Geometry check sheet. Reference: the model listing, model coordinates, mm. A direction names the side the tool comes from. Round coordinates to 2 decimals unless told otherwise and drop trailing zeros. Order: outer loops, then holes, each group sorted by start corner. A loop starts at its lowest first (then second) coordinate and runs counter-clockwise, first axis right, second up.
```python
from build123d import *

# Parameters (mm, degrees)
F1_DEPTH = 20
F2_R     = 75
F3_DEPTH = 20.001
F4_R     = 5
F5_DEPTH = 20.001
F6_DEPTH = 25
F7_T     = -5


with BuildPart() as f1:
    # F0 (on Top) → F1 (new body)
    with BuildSketch(Plane.XY):
        Polygon((86.6025403784, -150), (173.2050807569, 0), (86.6025403784, 150), (-86.6025403784, 150), (-173.2050807569, 0), (-86.6025403784, -150), align=None)
    extrude(amount=F1_DEPTH)

    # F2 (on face) → F3 (cut, through all)
    with BuildSketch(Plane.XY.offset(20)):
        Circle(F2_R)
    extrude(amount=-F3_DEPTH, mode=Mode.SUBTRACT)

    # F4 (on face) → F5 (cut, through all)
    with BuildSketch(Plane.XY.offset(20)):
        with Locations((75, 129.9038105677)):
            Circle(F4_R)
        with Locations((-75, -129.9038105677)):
            Circle(F4_R)
        with Locations((-150, 0)):
            Circle(F4_R)
        with Locations((150, 0)):
            Circle(F4_R)
        with Locations((75, -129.9038105677)):
            Circle(F4_R)
    extrude(amount=-F5_DEPTH, mode=Mode.SUBTRACT)

    # F4 (on face) → F6 (cut)
    with BuildSketch(Plane.XY.offset(20)):
        with Locations((-75, 129.9038105677)):
            Circle(F4_R)
        with Locations((75, 129.9038105677)):
            Circle(F4_R)
        with Locations((-75, -129.9038105677)):
            Circle(F4_R)
        with Locations((-150, 0)):
            Circle(F4_R)
        with Locations((150, 0)):
            Circle(F4_R)
        with Locations((75, -129.9038105677)):
            Circle(F4_R)
    extrude(amount=-F6_DEPTH, mode=Mode.SUBTRACT)

    # F7
    f7_openings = [f1.faces().sort_by_distance(p)[0] for p in [
        (0, -145.417424, 0),
    ]]
    offset(amount=F7_T, openings=f7_openings)


solid = f1.part
```
(1) Draft check along Y on faces 3 (the flat face through (129.298, -76.05, 9.86)), 4 (the flat face through (23.3, 71.5, 0)), 5 (the cylindrical face through (-9.764, 74.362, 10.14)). Enter one of: released by +Y, released by -Y, zero draft, split by the parting line, or undercut.
Returned:
face 3: released by -Y
face 4: zero draft
face 5: undercut
(2) Material ranges on line 1 (X direction, y = -59, z = 2.75); line 2 (Y direction, x = -7, z = 4.75); line 3 (X direction, y = 53, z = 10.25), recorded low to high.
Returned:
line 1: x = -139.14 to -133.37, -54.03 to -46.3, 46.3 to 54.03, 133.37 to 139.14
line 2: y = -150 to -145, -79.69 to -74.67, 74.67 to 79.69, 145 to 150
line 3: x = -142.61 to -136.83, -59.92 to -53.07, 53.07 to 59.92, 136.83 to 142.61
(3) Sectioned sample at A-A, the plane z = 5. Give the number of separate pieces and of enclosed holes in the cut face, and give its area (3 significant figures).
Returned:
separate pieces: 8
enclosed holes: 8
area: 8,960 mm2
(4) Depth check by flat-ended pin: P1, Ø4, axis at y = -108.5, z = 2, coming from the -X side; P2, Ø3, axis at x = 131.5, z = 3.5, coming from the +Y side; P3, Ø1, axis at y = 119.5, z = 10, coming from the -X side; P4, Ø16, axis at x = -75, y = -129.9, coming from the +Z side. Enter the tip coordinate at first touch or a pass-through.
Returned:
P1: stops at x = -111.72
P2: stops at y = 74.83
P3: stops at x = -104.5
P4: stops at z = 20
(5) Sectioned sample at C-C, the plane y = 47.5. Record the cut outline in (x, z), and give its area (3 significant figures).
Returned:
outline: (-145.78, 0) - (-140.01, 0) - (-140.01, 15) - (-64.37, 15) - (-64.37, 0) - (-58.04, 0) - (-58.04, 20) - (-145.78, 20) - close; (58.04, 0) - (64.37, 0) - (64.37, 15) - (140.01, 15) - (140.01, 0) - (145.78, 0) - (145.78, 20) - (58.04, 20) - close
area: 1,240 mm2
(6) Set-up check for faces 1 (the cylindrical face through (67.63, 136.66, 7.6)), 2 (the flat face through (70, 128, 0)): record each of +Z, -Z, +X, -X, +Y, -Y from which the full face is reachable in a straight line by a thin tool's end or side.
Returned:
face 1: -Z
face 2: -Z, +X, -X, +Y, -Y
(7) Sectioned sample at B-B, the plane x = -150. Record the cut outline in (y, z), and give its area (3 significant figures).
Returned:
outline: (-40.19, 0) - (-30.19, 0) - (-30.19, 15) - (-10, 15) - (-10, 0) - (-5, 0) - (-5, 20) - (-40.19, 20) - close; (5, 0) - (10, 0) - (10, 15) - (30.19, 15) - (30.19, 0) - (40.19, 0) - (40.19, 20) - (5, 20) - close
area: 802 mm2
